The model under review builds one solid part; all positions refer to its coordinate system, in mm. Face numbers are marked on the shaded views. A direction names the side the tool comes from. Give positions to 0.01 mm unless a question says otherwise; leave off trailing zeros. Order: outer loops, then holes, each group sorted by start corner. A loop starts at its lowest first (then second) coordinate and runs counter-clockwise, first axis right, second up.
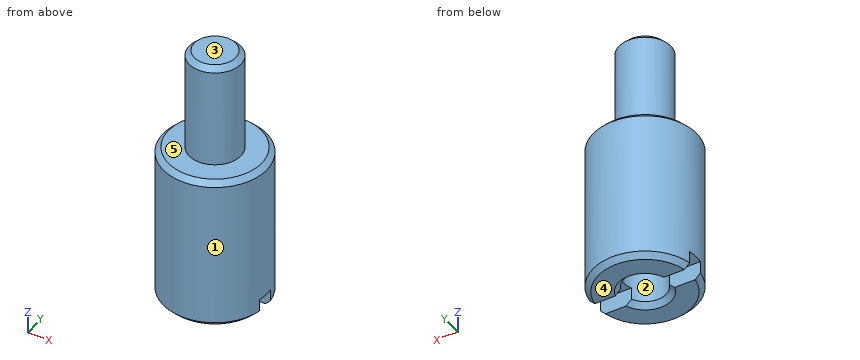
Autodesk Inventor part; units mm, degrees
ref_plane "YZ Plane" through (0, 0, 0) normal (1, 0, 0) x (0, 1, 0)
ref_plane "XZ Plane" through (0, 0, 0) normal (0, 1, 0) x (-1, 0, 0)
ref_plane "XY Plane" through (0, 0, 0) normal (0, 0, 1) x (1, 0, 0)
sketch "Sketch1" plane through (0, 0, 0) normal (0, 1, 0) x (-1, 0, 0)
  line L0 (0, 0) -> (-3, 0)
  line L1 (-3, 0) -> (-3, 9)
  line L2 (-3, 9) -> (-1.5, 9)
  line L3 (-1.5, 9) -> (-1.5, 15)
  line L4 (-1.5, 15) -> (0, 15)
  line L5 (0, 15) -> (0, 0)
  dimension "d1" = 6
  dimension "d2" = 9
  dimension "d3" = 3
  dimension "d4" = 6
revolve "Revolution1" add sketch "Sketch1" angle 360 about axis through (0, 0, 15) along (0, 0, -1)
sketch "Sketch2" plane through (0, 0, 0) normal (0, 0, -1) x (-1, 0, 0)
  line L0 (-3, -0.5) -> (3, -0.5)
  line L1 (3, -0.5) -> (3, 0.5)
  line L2 (3, 0.5) -> (-3, 0.5)
  line L3 (-3, 0.5) -> (-3, -0.5)
  line L4 (-3, -0.5) -> (3, 0.5) construction
  line L5 (3, -0.5) -> (-3, 0.5) construction
  circle A0 centre (0, 0) radius 3
  dimension "d6" = 1
extrude "Extrusion1" cut sketch "Sketch2" against normal blind 1 contours L3 A0 L0 | A0 L2 L0 | L3 L2 A0 | A0 L1 L0 | A0 L2 L1
hole "Hole1" at (0, 0, 0) direction (0, 0, 1) diameter 2.459 depth 6
thread "Thread1"
chamfer "Chamfer1" distance 0.3 angle 45 7 edges at (-3, 0, 9) (0, 3, 0) (0, -3, 0) (0, -1.2295, 0) (-0.6697, 1.0311, 0) (0.6697, 1.0311, 0) (-1.5, 0, 15)
properties part number "BRU-309S" material "Stainless Steel AISI 304"
Item 1: For line 1 (Y direction, x = 0.1, z = 4); line 2 (Z direction, x = 0.3, y = -1.75), list the stretches that pass through material, from the lowest coordinate up.
Values found:
line 1: y = -3 to -1.23, 1.23 to 3
line 2: z = 0 to 9
Item 2: Take a section at C-C (z = 10.5). Give the boundary of the cut face in (x, y), and give its area (3 significant figures).
Values found:
outline: circle Ø3 at (0, 0)
area: 7.07 mm2
Item 3: Clearance check with flat-ended pins moving along their axes: pin 1 Ø0.8 at (x, y) = (-1.5, 0) entering from -Z; pin 2 Ø1.1 at (x, z) = (2, 0.5) entering from -Y; pin 3 Ø1.2 at (x, y) = (0.5, 0) entering from -Z. State where each tip first meets the part, or that it passes through.
Values found:
pin 1: stops at z = 1
pin 2: stops at y = -2.63
pin 3: stops at z = 6
Item 4: Take a section at B-B (x = 0). Give the boundary of the cut face in (y, z).
Values found:
outline: (-3, 0.3) - (-2.7, 0) - (-1.53, 0) - (-1.23, 0.3) - (-1.23, 6) - (1.23, 6) - (1.23, 0.3) - (1.53, 0) - (2.7, 0) - (3, 0.3) - (3, 8.7) - (2.7, 9) - (1.5, 9) - (1.5, 14.7) - (1.2, 15) - (-1.2, 15) - (-1.5, 14.7) - (-1.5, 9) - (-2.7, 9) - (-3, 8.7) - close
Item 5: Take a section at A-A (y = 0). Give the boundary of the cut face in (x, z).
Values found:
outline: (-3, 1) - (-1.23, 1) - (-1.23, 6) - (1.23, 6) - (1.23, 1) - (3, 1) - (3, 8.7) - (2.7, 9) - (1.5, 9) - (1.5, 14.7) - (1.2, 15) - (-1.2, 15) - (-1.5, 14.7) - (-1.5, 9) - (-2.7, 9) - (-3, 8.7) - close
Item 6: For the marked faces 4 and 5, list the 3-axis set-ups (+Z, -Z, +X, -X, +Y, -Y) from which the entire face can be reached by the end or side of a thin tool; tool diameter is ignored.
Values found:
face 4: -Z, +X, -X, +Y, -Y
face 5: +Z
Item 7: Draft analysis for pull direction X (two halves, no side actions). For the marked faces 1, 2 and 3, state which applies: released by +X, released by -X, zero draft, split by the parting line, or undercut.
Values found:
face 1: split by the parting line
face 2: undercut
face 3: zero draft
Item 8: Take a section at D-D (z = 7). Give the boundary of the cut face in (x, y), and give its area (3 significant figures).
Values found:
outline: circle Ø6 at (0, 0)
area: 28.3 mm2
